Verification items for the finished model (mm, model axes). A direction names the side the tool comes from. Coordinates: 2 decimals unless noted, no trailing zeros. Return JSON: item names as keys, results as strings.
```python
from build123d import *

# Parameters (mm, degrees)
SKETCH_R     = 2.5
PAD_DEPTH    = 460
SKETCH001_W  = 70
SKETCH001_H  = 25
POCKET_DEPTH = 14.5


with BuildPart() as part:
    # Sketch → Pad (new body)
    with BuildSketch(Plane.YZ):
        with BuildLine():
            Line((-43.1, 0), (-37.459288, 9.77))
            Line((-37.459288, 9.77), (-60, 9.77))
            Line((-60, 9.77), (-60, 41.5))
            Line((-60, 41.5), (-39.5, 41.5))
            Line((-39.5, 41.5), (-39.5, 32.5))
            Line((-39.5, 32.5), (-45, 32.5))
            Line((-45, 32.5), (-45, 25.5))
            Line((-45, 25.5), (-23.75, 25.5))
            Line((-23.75, 25.5), (-23.75, 32.5))
            Line((-23.75, 32.5), (-27.5, 32.5))
            Line((-27.5, 32.5), (-27.5, 40))
            Line((-27.5, 40), (-5, 40))
            Line((-5, 40), (-5, 32.5))
            Line((-5, 32.5), (-8.75, 32.5))
            Line((-8.75, 32.5), (-8.75, 25.5))
            Line((-8.75, 25.5), (10.75, 25.5))
            Line((10.75, 25.5), (10.75, 32.5))
            Line((7, 32.5), (10.75, 32.5))
            Line((7, 32.5), (7, 40))
            Line((7, 40), (29.5, 40))
            Line((29.5, 40), (29.5, 32.5))
            Line((29.5, 32.5), (25.75, 32.5))
            Line((25.75, 32.5), (25.75, 25.5))
            Line((25.75, 25.5), (47, 25.5))
            Line((47, 25.5), (47, 32.5))
            Line((47, 32.5), (41.5, 32.5))
            Line((41.5, 32.5), (41.5, 41.5))
            Line((41.5, 41.5), (60, 41.5))
            Line((60, 41.5), (60, 9.77))
            Line((60, 9.77), (33.859288, 9.77))
            Line((33.859288, 9.77), (39.5, 0))
            Line((39.5, 0), (21, 0))
            Line((19.843853, 11), (21, 0))
            ThreePointArc((19.843853, 11), (17.886929, 14.396937), (14.25, 15.860317))
            Line((10.25, 16), (14.25, 15.860317))
            Line((10.25, 16), (10.25, 17))
            Line((10.25, 17), (-10.25, 17))
            Line((-10.25, 17), (-10.25, 16))
            Line((-14.25, 15.860317), (-10.25, 16))
            ThreePointArc((-14.25, 15.860317), (-18.255593, 14.588138), (-20.443853, 11))
            Line((-21.6, 0), (-20.443853, 11))
            Line((-21.6, 0), (-43.1, 0))
        make_face()
        with Locations((36, 19.3)):
            Circle(SKETCH_R, mode=Mode.SUBTRACT)
        with Locations((-36, 19.3)):
            Circle(SKETCH_R, mode=Mode.SUBTRACT)
    extrude(amount=PAD_DEPTH)

    # Sketch001 → Pocket (cut)
    with BuildSketch(Plane(origin=(0, 0, 40), x_dir=(0, -1, 0), z_dir=(0, 0, 1))):
        with Locations((0, 12.5)):
            Rectangle(SKETCH001_W, SKETCH001_H)
        with Locations((0, 447.5)):
            Rectangle(SKETCH001_W, SKETCH001_H)
    extrude(amount=-POCKET_DEPTH, mode=Mode.SUBTRACT)


solid = part.part
```
Q1. Material ranges on line 1 along Y through (x, z) = (438.5, 19); line 2 along Y through (x, z) = (94.5, 28); line 3 along Z through (x, y) = (100.5, -36), recorded low to high.
Values:
{"line 1": "-60 to -38.48, -33.52 to 33.52, 38.48 to 60", "line 2": "-60 to -45, -23.75 to -8.75, 10.75 to 25.75, 47 to 60", "line 3": "0 to 16.8, 21.8 to 25.5"}
Q2. Tool access check on faces 4 (the face through (25, 18, 33)), 5 (the face through (435, 18, 33)), 6 (the face through (226.78, -21.03, 5.42)), 7 (the face through (227, -16, 40)). Record the directions out of +Z, -Z, +X, -X, +Y, -Y that give a thin tool (end or side, any length) a straight path to the whole face; none if there is none.
Values:
{"face 4": "+Z, -X", "face 5": "+Z, +X", "face 6": "-Z, +X, -X", "face 7": "+Z, +X, -X"}
Q3. Go/stop test with flat-tipped pins: pin 1 (18 mm diameter, centred on x = 185, y = 23, fed in from +Z); pin 2 (8 mm diameter, centred on x = 133.5, y = -33.5, fed in from +Z); pin 3 (4 mm diameter, centred on x = 324, y = 9.5, fed in from -Z). Record where each tip stops, or that it passes through.
Values:
{"pin 1": "z = 40", "pin 2": "z = 25.5", "pin 3": "z = 15.96"}
Q4. Cross-section at A-A, the plane x = 276.5. State how many separate pieces and enclosed holes the cut face has, and give its area (3 significant figures).
Values:
{"separate pieces": "1", "enclosed holes": "2", "area": "3,030 mm^2"}
Q5. Draft check along Z on faces 1 (the face through (227, 29.5, 36)), 2 (the face through (226.78, 36.64, 4.95)), 3 (the face through (227, -50, 41.5)). Enter one of: pulls with the +Z half, pulls with the -Z half, needs draft (parallel to the pull), parting line crosses it, or undercut.
Values:
{"face 1": "needs draft", "face 2": "undercut", "face 3": "pulls with the +Z half"}
